from build123d import *

# Parameters (mm, degrees)
F0_W     = 7.04
F0_H     = 8.55
F1_DEPTH = 6.8
F3_DEPTH = 7.04
F4_W     = 2.92
F4_H     = 4.15
F5_DEPTH = 5
F6_R     = 1.35
F7_DEPTH = 1
F8_R     = 0.4
F9_DEPTH = 3.65


with BuildPart() as f1:
    # F0 (on Front) → F1 (new body)
    with BuildSketch(Plane.XZ):
        with Locations((3.52, 4.275)):
            Rectangle(F0_W, F0_H)
    extrude(amount=F1_DEPTH)

    # F2 (on face) → F3 (cut, through all)
    with BuildSketch(Plane.YZ.offset(7.04)):
        Polygon((-6.8, 8.55), (-6.8, 4.75), (-5.4, 8.55), align=None)
        Polygon((0, 4.75), (0, 8.55), (-1.4, 8.55), align=None)
    extrude(amount=-F3_DEPTH, mode=Mode.SUBTRACT)

    # F4 (on face) → F5 (cut)
    with BuildSketch(Plane.XZ.offset(6.8)):
        with Locations((1.76, 2.675)):
            Rectangle(F4_W, F4_H)
        with Locations((5.28, 2.675)):
            Rectangle(F4_W, F4_H)
    extrude(amount=-F5_DEPTH, mode=Mode.SUBTRACT)

    # F6 (on face) → F7 (cut)
    with BuildSketch(Plane.XY.offset(8.55)):
        with Locations((1.76, -3.4)):
            Circle(F6_R)
        with Locations((5.28, -3.4)):
            Circle(F6_R)
    extrude(amount=-F7_DEPTH, mode=Mode.SUBTRACT)

    # F8 (on face) → F9 (join)
    with BuildSketch(Plane(origin=(0, 0, 0), x_dir=(1, 0, 0), z_dir=(0, 0, -1))):
        with Locations((1.76, 3.4)):
            Circle(F8_R)
        with Locations((5.28, 3.4)):
            Circle(F8_R)
    extrude(amount=F9_DEPTH)


solid = f1.part
Input: part model. Units: mm. Frame: model coordinates. A direction names the side the tool comes from. Coordinates: 2 decimals unless noted, no trailing zeros. Write each loop counter-clockwise with the first axis right and the second up, starting at its lowest first coordinate (ties: lowest second). Pieces come first, ordered by that corner, then holes. Notation, with made-up numbers: M -15.5,67.25 L -7.5,67.25 A34 ccw -7.5,97.25 Z; hole C 71,-11.5 d5. An arc over 180 degrees is marked long. Answer as a JSON object with one key per item and string values. Group by question number.
(1) Section D-D on z = -1.75. Output: boundary loops of the cut face in (x, y).
(2) Section A-A on z = 1.25. Output: boundary loops of the cut face in (x, y), plus the area to 3 significant figures.
(3) Section C-C on y = -3.4. Output: boundary loops of the cut face in (x, z).
(4) Section B-B on x = 5.28. Output: boundary loops of the cut face in (y, z).
(5) Mould query, pull axis Z, two halves, no side actions, for faces 5 (the face through (3, 0, 2)), 6 (the face through (5, -3, 7.55)), 7 (the face through (3.82, -4, 3)). Classes: pulls with the +Z half, pulls with the -Z half, needs draft (parallel to the pull), parting line crosses it, or undercut.
(6) Set-up query: faces 1 (the face through (2.14, -3.52, -1.8)), 2 (the face through (3.57, -0.71, 6.68)), 3 (the face through (3.048, -2.994, 8.057)), 4 (the face through (3.22, -4, 3)). Return all of +Z, -Z, +X, -X, +Y, -Y with unobstructed straight access to the full face (end or side cutting, diameter ignored); none if empty.
(7) Contact query for a flat-ended pin moving along its axis: P1, Ø1.5, axis at x = 5.5, z = 2, coming from the -Y side. Output: stop coordinate, or through.
(8) Ray query, line 1 along X through (y, z) = (-2.25, 3); line 2 along Z through (x, y) = (4.5, -4); line 3 along Z through (x, y) = (6.5, -2.75). Return the intervals inside material, ascending. Write a range as [from, to].
Result set:
{
 "1": {"outline": "C 1.76,-3.4 d0.8; C 5.28,-3.4 d0.8"},
 "2": {"outline": "M 0,-6.8 L 0.3,-6.8 L 0.3,-1.8 L 3.22,-1.8 L 3.22,-6.8 L 3.82,-6.8 L 3.82,-1.8 L 6.74,-1.8 L 6.74,-6.8 L 7.04,-6.8 L 7.04,0 L 0,0 Z", "area": "18.7 mm2"},
 "3": {"outline": "M 0,0 L 1.36,0 L 1.36,-3.65 L 2.16,-3.65 L 2.16,0 L 4.88,0 L 4.88,-3.65 L 5.68,-3.65 L 5.68,0 L 7.04,0 L 7.04,8.55 L 6.63,8.55 L 6.63,7.55 L 3.93,7.55 L 3.93,8.55 L 3.11,8.55 L 3.11,7.55 L 0.41,7.55 L 0.41,8.55 L 0,8.55 Z; hole M 0.3,0.6 L 3.22,0.6 L 3.22,4.75 L 0.3,4.75 Z; hole M 3.82,0.6 L 6.74,0.6 L 6.74,4.75 L 3.82,4.75 Z"},
 "4": {"outline": "M -6.8,0 L -3.8,0 L -3.8,-3.65 L -3,-3.65 L -3,0 L 0,0 L 0,4.75 L -1.4,8.55 L -2.05,8.55 L -2.05,7.55 L -4.75,7.55 L -4.75,8.55 L -5.4,8.55 L -6.8,4.75 L -1.8,4.75 L -1.8,0.6 L -6.8,0.6 Z"},
 "5": {"face 5": "needs draft", "face 6": "pulls with the +Z half", "face 7": "undercut"},
 "6": {"face 1": "-Z", "face 2": "+Z, +X, -X, +Y", "face 3": "+Z", "face 4": "-Y"},
 "7": {"P1": "stops at y = -1.8"},
 "8": {"line 1": "x = [0, 0.3], [3.22, 3.82], [6.74, 7.04]", "line 2": "z = [0, 0.6], [4.75, 7.55]", "line 3": "z = [0, 0.6], [4.75, 8.55]"}
}
